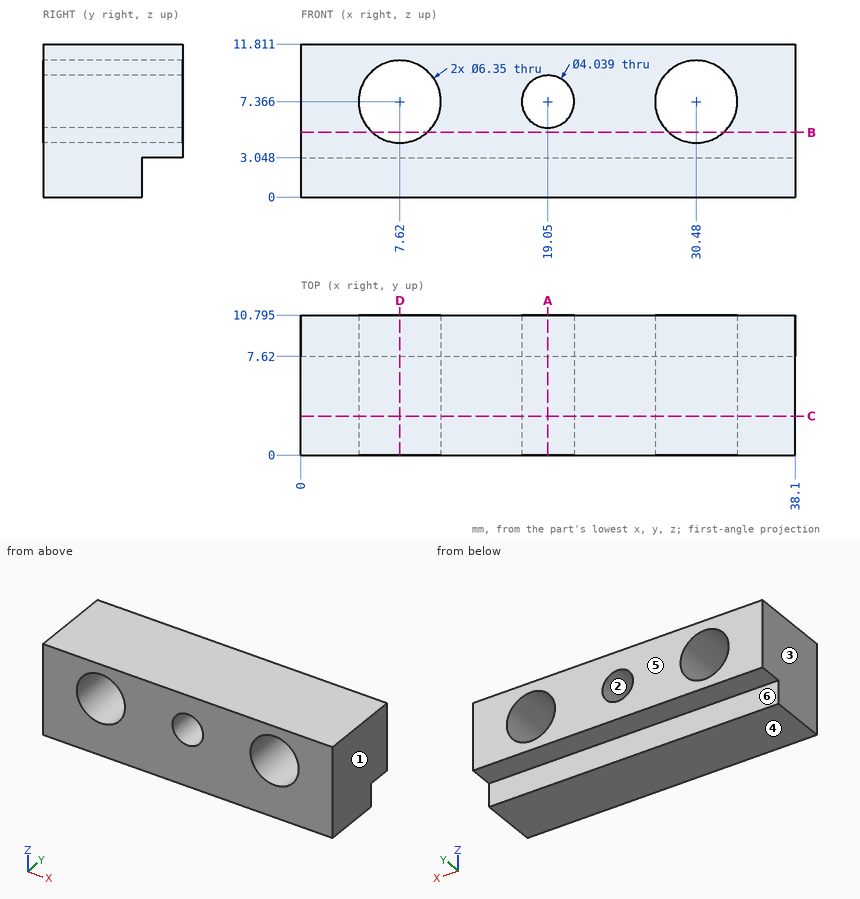
For this review, use the dimensioned drawing (mm, ordinates from the lowest corner) and the shaded views. A direction names the side the tool comes from. Give positions to 0.01 mm unless a question says otherwise; leave off trailing zeros. Order: outer loops, then holes, each group sorted by start corner. A loop starts at its lowest first (then second) coordinate and runs counter-clockwise, first axis right, second up. Notation, with made-up numbers: M 63,-18 L 85,-18 A26 cw 85,13 Z; hole C 6.25,81.5 d11. An arc over 180 degrees is marked long. Use one line per item in the form item = value. Start each with the question number.
Item 1: We need section A-A on x = 19.05. Give the boundary of the cut face in (y, z) (1 decimal).
Item 2: For the marked faces 5 and 6, list the 3-axis set-ups (+Z, -Z, +X, -X, +Y, -Y) from which the entire face can be reached by the end or side of a thin tool; tool diameter is ignored.
Item 3: We need section B-B on z = 5. Give the boundary of the cut face in (x, y) (1 decimal), plus the area to 3 significant figures.
Item 4: We need section C-C on y = 3. Give the number of separate pieces and of enclosed holes in the cut face, plus the area to 3 significant figures.
Item 5: The part is to be moulded in two halves that separate along X. For the marked faces 1, 2, 3 and 4, say which applies: pulls with the +X half, pulls with the -X half, needs draft (parallel to the pull), parting line crosses it, or undercut.
Item 6: Insertion check: pin 1 Ø2.5 at (x, y) = (26, 9) entering from -Z. The pin has a flat end and moves straight along its axis. Give the tip position at first contact, or say it passes through.
Item 7: We need section D-D on x = 7.62. Give the boundary of the cut face in (y, z) (1 decimal).
Item 8: To check wall thickness, follow line 1 along Z through (x, y) = (7.62, 6); line 2 along X through (y, z) = (8.75, 9.5); line 3 along X through (y, z) = (1.25, 9.75) (1 decimal). State the ranges of each line that lie inside material, in increasing order. Write a range as from..to.
Completed:
q1.outline = M 0,0 L 7.6,0 L 7.6,3 L 10.8,3 L 10.8,5.3 L 0,5.3 Z; M 0,9.4 L 10.8,9.4 L 10.8,11.8 L 0,11.8 Z
q2.face_5 = +Z, -Z, +X, -X, +Y
q2.face_6 = -Z, +X, -X, +Y
q3.outline = M 0,0 L 5.5,0 L 5.5,10.8 L 0,10.8 Z; M 9.7,0 L 28.4,0 L 28.4,10.8 L 9.7,10.8 Z; M 32.6,0 L 38.1,0 L 38.1,10.8 L 32.6,10.8 Z
q3.area = 320 mm²
q4.separate_pieces = 1
q4.enclosed_holes = 3
q4.area = 374 mm²
q5.face_1 = pulls with the +X half
q5.face_2 = undercut
q5.face_3 = pulls with the -X half
q5.face_4 = needs draft
q6.pin_1 = 3.05
q7.outline = M 0,0 L 7.6,0 L 7.6,3 L 10.8,3 L 10.8,4.2 L 0,4.2 Z; M 0,10.5 L 10.8,10.5 L 10.8,11.8 L 0,11.8 Z
q8.line_1 = 0..4.19, 10.54..11.81
q8.line_2 = 0..5.27, 9.97..28.13, 32.83..38.1
q8.line_3 = 0..5.5, 9.7..28.4, 32.6..38.1
